from build123d import *

# Parameters (mm, degrees)
SKETCH1_W           = 304.8
SKETCH1_H           = 304.8
BOSS_EXTRUDE1_DEPTH = 2.778125
SKETCH2_W           = 304.8
SKETCH2_H           = 19.05
CUT_EXTRUDE1_DEPTH  = 3.778125
CUT_EXTRUDE2_DEPTH  = 3.778125
SKETCH4_R           = 1.7526
CUT_EXTRUDE3_DEPTH  = 3.778125
SKETCH5_W           = 9.525
SKETCH5_H           = 266.7
CUT_EXTRUDE4_DEPTH  = 3.778125
FILLET1_R           = 2.54


with BuildPart() as part:
    # Sketch1 → Boss-Extrude1 (new body)
    with BuildSketch(Plane(origin=(0, 0, 0), x_dir=(1, 0, 0), z_dir=(0, 1, 0))):
        with Locations((152.4, 152.4)):
            Rectangle(SKETCH1_W, SKETCH1_H)
    extrude(amount=BOSS_EXTRUDE1_DEPTH)

    # Sketch2 → Cut-Extrude1 (cut, through all)
    with BuildSketch(Plane(origin=(0, 2.778125, 0), x_dir=(1, 0, 0), z_dir=(0, 1, 0))):
        with Locations((152.4, 9.525)):
            Rectangle(SKETCH2_W, SKETCH2_H)
        with Locations((152.4, 295.275)):
            Rectangle(SKETCH2_W, SKETCH2_H)
    extrude(amount=-CUT_EXTRUDE1_DEPTH, mode=Mode.SUBTRACT)

    # Sketch3 → Cut-Extrude2 (cut, through all)
    with BuildSketch(Plane(origin=(0, 2.778125, 0), x_dir=(1, 0, 0), z_dir=(0, 1, 0))):
        Polygon((50.8, 285.75), (0, 285.75), (0, 228.6), (9.525, 228.6), (9.525, 269.875), (50.8, 269.875), align=None)
        Polygon((0, 19.05), (0, 76.2), (9.525, 76.2), (9.525, 34.925), (50.8, 34.925), (50.8, 19.05), align=None)
    extrude(amount=-CUT_EXTRUDE2_DEPTH, mode=Mode.SUBTRACT)

    # Sketch4 → Cut-Extrude3 (cut, through all)
    with BuildSketch(Plane(origin=(0, 2.778125, 0), x_dir=(1, 0, 0), z_dir=(0, 1, 0))):
        with Locations((12.7, 190.5762)):
            Circle(SKETCH4_R)
        with Locations((12.7, 114.3762)):
            Circle(SKETCH4_R)
    extrude(amount=-CUT_EXTRUDE3_DEPTH, mode=Mode.SUBTRACT)

    # Sketch5 → Cut-Extrude4 (cut, through all)
    with BuildSketch(Plane(origin=(0, 2.778125, 0), x_dir=(1, 0, 0), z_dir=(0, 1, 0))):
        with Locations((300.0375, 152.4)):
            Rectangle(SKETCH5_W, SKETCH5_H)
    extrude(amount=-CUT_EXTRUDE4_DEPTH, mode=Mode.SUBTRACT)

    # Fillet1
    fillet1_edges = [part.edges().sort_by_distance(p)[0] for p in [
        (295.275, 1.3890625, -19.05),
        (295.275, 1.3890625, -285.75),
        (50.8, 1.3890625, -285.75),
        (50.8, 1.3890625, -269.875),
        (9.525, 1.3890625, -269.875),
        (0, 1.3890625, -228.6),
        (50.8, 1.3890625, -19.05),
        (0, 1.3890625, -76.2),
        (9.525, 1.3890625, -76.2),
        (9.525, 1.3890625, -34.925),
        (50.8, 1.3890625, -34.925),
    ]]
    fillet(fillet1_edges, radius=FILLET1_R)


solid = part.part
Geometry: final body of the model. Coordinates: model frame, mm. Give positions to 0.01 mm unless a question says otherwise; leave off trailing zeros. Loops run counter-clockwise (first coordinate to the right, second up) from the corner with the lowest first, then second, coordinate; pieces in that order, holes last. Notation, with made-up numbers: (-19, 31) -> (6, 31) arc R34 ccw to (6, 61) -> close; hole circle Ø11 at (-32, -33). An arc over 180 degrees is marked (long way). Put each result on its own line as item: value.
1. Ray query, line 1 along Z through (x, y) = (12.7, 2.1) (3 decimals); line 2 along X through (y, z) = (2.4, -74) (3 decimals); line 3 along X through (y, z) = (2.15, -274) (3 decimals). Return the intervals inside material, ascending. Write a range as [from, to].
Taken from the geometry:
line 1: z = [-269.875, -192.329], [-188.824, -116.129], [-112.624, -34.925]
line 2: x = [9.502, 295.275]
line 3: x = [50.8, 295.275]
2. Cut plane B-B (z = -63.5). Return the cut outline in (x, y) (3 decimals), plus the area to 3 significant figures.
Taken from the geometry:
outline: (9.525, 0) -> (295.275, 0) -> (295.275, 2.778) -> (9.525, 2.778) -> close
area: 794 mm2
3. Pin query (flat end, axial travel): P1, Ø1.4, axis at y = 2, z = -277, coming from the -X side; P2, Ø0.8, axis at x = 35, y = 1, coming from the +Z side (3 decimals); P3, Ø1.4, axis at y = 1.5, z = -239.5, coming from the -X side (3 decimals); P4, Ø3, axis at x = 12.7, z = -190.58, coming from the -Y side. Return the tip coordinate at first contact, or that it passes through.
Taken from the geometry:
P1: stops at x = 50.8
P2: stops at z = -34.925
P3: stops at x = 9.525
P4: passes through
4. Cut plane A-A (y = 1.45). Return the cut outline in (x, z) (3 decimals), plus the area to 3 significant figures.
Taken from the geometry:
outline: (0, -226.06) arc R2.54 ccw to (2.54, -228.6) -> (9.525, -228.6) -> (9.525, -267.335) arc R2.54 ccw to (12.065, -269.875) -> (48.26, -269.875) arc R2.54 cw to (50.8, -272.415) -> (50.8, -283.21) arc R2.54 ccw to (53.34, -285.75) -> (292.735, -285.75) arc R2.54 ccw to (295.275, -283.21) -> (295.275, -21.59) arc R2.54 ccw to (292.735, -19.05) -> (53.34, -19.05) arc R2.54 ccw to (50.8, -21.59) -> (50.8, -32.385) arc R2.54 cw to (48.26, -34.925) -> (12.065, -34.925) arc R2.54 ccw to (9.525, -37.465) -> (9.525, -73.66) arc R2.54 cw to (6.985, -76.2) -> (2.54, -76.2) arc R2.54 ccw to (0, -78.74) -> close; hole circle Ø3.505 at (12.7, -190.576); hole circle Ø3.505 at (12.7, -114.376)
area: 76,300 mm2
